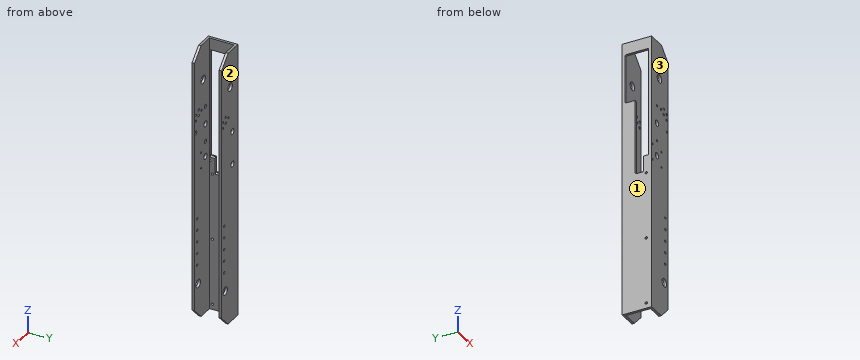
```python
from build123d import *

# Parameters (mm, degrees)
BOSS_EXTRUDE1_DEPTH                                 = 700
CUT_EXTRUDE1_DEPTH                                  = 706.00443261
CHAMFER1_SIZE                                       = 30
SKETCH4_R                                           = 10.5
CUT_EXTRUDE2_DEPTH                                  = 708.990112925
SKETCH5_R                                           = 7.5
CUT_EXTRUDE3_DEPTH                                  = 708.990112925
CHAMFER2_SIZE                                       = 3
FILLET1_R                                           = 3
SKETCH6_R                                           = 3
TENSIONER_HOLES_DEPTH                               = 708.990112925
CSK_FOR_M5_COUNTERSUNK_FLAT_HEAD_SCREW1_D           = 5.8
CSK_FOR_M5_COUNTERSUNK_FLAT_HEAD_SCREW1_DEPTH       = 12
CSK_FOR_M5_COUNTERSUNK_FLAT_HEAD_SCREW1_CSINK_D     = 10.4
CSK_FOR_M5_COUNTERSUNK_FLAT_HEAD_SCREW1_CSINK_ANGLE = 90
CSK_FOR_M5_COUNTERSUNK_FLAT_HEAD_SCREW1_TIP         = 1.742495795
SKETCH11_R                                          = 3
CUT_EXTRUDE4_DEPTH                                  = 10
SKETCH13_R                                          = 2.55
CUT_EXTRUDE5_DEPTH                                  = 10


with BuildPart() as part:
    # Sketch1 → Boss-Extrude1 (new body)
    with BuildSketch(Plane.XY):
        Polygon((0, -37.5), (0, 37.5), (75, 37.5), (75, 31.15), (6.35, 31.15), (6.35, -31.15), (75, -31.15), (75, -37.5), align=None)
    extrude(amount=BOSS_EXTRUDE1_DEPTH)

    # Sketch3 → Cut-Extrude1 (cut, through all)
    with BuildSketch(Plane.ZY):
        Polygon((670.5, -30), (545.5, -30), (395.5, -30), (395.5, -16.85), (355, -16.85), (355, 4.15), (460, 4.15), (545.5, 4.15), (545.5, 30), (670.5, 30), align=None)
    extrude(amount=-CUT_EXTRUDE1_DEPTH, mode=Mode.SUBTRACT)

    # Chamfer1
    chamfer1_edges = [part.edges().sort_by_distance(p)[0] for p in [
        (75, -34.325, 0),
        (75, 34.325, 700),
        (75, -34.325, 700),
        (75, 34.325, 0),
    ]]
    chamfer(chamfer1_edges, length=CHAMFER1_SIZE)

    # Sketch4 → Cut-Extrude2 (cut, through all)
    with BuildSketch(Plane(origin=(0, 37.5, 0), x_dir=(1, 0, 0), z_dir=(0, 1, 0))):
        with Locations(Location((36, -608, 0), (0, 0, 270))):
            Circle(SKETCH4_R)
        with Locations(Location((58.5, -92, 0), (0, 0, 270))):
            Circle(SKETCH4_R)
    extrude(amount=-CUT_EXTRUDE2_DEPTH, mode=Mode.SUBTRACT)

    # Sketch5 → Cut-Extrude3 (cut, through all)
    with BuildSketch(Plane.XZ.offset(37.5)):
        with Locations(Location((25, 487.498060398, 0), (0, 0, 270))):
            Circle(SKETCH5_R)
        with Locations(Location((24.951834767, 403.39807419, 0), (0, 0, 270))):
            Circle(SKETCH5_R)
    extrude(amount=-CUT_EXTRUDE3_DEPTH, mode=Mode.SUBTRACT)

    # Chamfer2
    chamfer2_edges = [part.edges().sort_by_distance(p)[0] for p in [
        (6.35, -23.425, 395.5),
        (6.35, -6.35, 355),
        (6.35, 17.075, 545.5),
    ]]
    chamfer(chamfer2_edges, length=CHAMFER2_SIZE)

    # Fillet1
    fillet1_edges = [part.edges().sort_by_distance(p)[0] for p in [
        (1.675, 4.15, 355),
        (1.675, -16.85, 355),
        (1.675, -30, 395.5),
        (1.675, 30, 545.5),
        (3.175, 30, 670.5),
        (3.175, -30, 670.5),
    ]]
    fillet(fillet1_edges, radius=FILLET1_R)

    # Sketch6 → tensioner holes (cut, through all)
    with BuildSketch(Plane(origin=(0, 37.5, 0), x_dir=(1, 0, 0), z_dir=(0, 1, 0))):
        with Locations(Location((69, -517.498060398, 0), (0, 0, 270))):
            Circle(SKETCH6_R)
        with Locations(Location((69, -532.498060398, 0), (0, 0, 270))):
            Circle(SKETCH6_R)
        with Locations(Location((56.009618943, -524.998060398, 0), (0, 0, 270))):
            Circle(SKETCH6_R)
        with Locations(Location((56.009618943, -539.998060398, 0), (0, 0, 270))):
            Circle(SKETCH6_R)
        with Locations(Location((63, -262, 0), (0, 0, 270))):
            Circle(SKETCH6_R)
        with Locations(Location((63, -232, 0), (0, 0, 270))):
            Circle(SKETCH6_R)
        with Locations(Location((63, -202, 0), (0, 0, 270))):
            Circle(SKETCH6_R)
        with Locations(Location((63, -172, 0), (0, 0, 270))):
            Circle(SKETCH6_R)
        with Locations(Location((63, -142, 0), (0, 0, 270))):
            Circle(SKETCH6_R)
        with Locations(Location((43.019237886, -532.498060398, 0), (0, 0, 270))):
            Circle(SKETCH6_R)
    extrude(amount=-TENSIONER_HOLES_DEPTH, mode=Mode.SUBTRACT)

    # CSK for M5 Countersunk Flat Head Screw1
    with Locations(Plane(origin=(0, -31.15, 0), x_dir=(-1, 0, 0), z_dir=(0, 1, 0))):
        with Locations((-25, 532.573060398), (-25, 442.423060398), (-70.075, 487.498060398)):
            CounterSinkHole(CSK_FOR_M5_COUNTERSUNK_FLAT_HEAD_SCREW1_D / 2, CSK_FOR_M5_COUNTERSUNK_FLAT_HEAD_SCREW1_CSINK_D / 2, depth=CSK_FOR_M5_COUNTERSUNK_FLAT_HEAD_SCREW1_DEPTH, counter_sink_angle=CSK_FOR_M5_COUNTERSUNK_FLAT_HEAD_SCREW1_CSINK_ANGLE)
            with Locations((0, 0, -(CSK_FOR_M5_COUNTERSUNK_FLAT_HEAD_SCREW1_DEPTH + CSK_FOR_M5_COUNTERSUNK_FLAT_HEAD_SCREW1_TIP / 2))):  # 118° drill point
                Cone(0, CSK_FOR_M5_COUNTERSUNK_FLAT_HEAD_SCREW1_D / 2, CSK_FOR_M5_COUNTERSUNK_FLAT_HEAD_SCREW1_TIP, mode=Mode.SUBTRACT)

    # Sketch11 → Cut-Extrude4 (cut)
    with BuildSketch(Plane.ZY):
        with Locations((350, -24)):
            Circle(SKETCH11_R)
        with Locations((13.5, -24)):
            Circle(SKETCH11_R)
        with Locations((181.75, -24)):
            Circle(SKETCH11_R)
    extrude(amount=-CUT_EXTRUDE4_DEPTH, mode=Mode.SUBTRACT)

    # Sketch13 → Cut-Extrude5 (cut)
    with BuildSketch(Plane.XZ.offset(37.5)):
        with Locations(Location((5.152844894, 423.197064064, 0), (0, 0, 270))):
            Circle(SKETCH13_R)
        with Locations(Location((5.152844894, 383.599084317, 0), (0, 0, 270))):
            Circle(SKETCH13_R)
        with Locations(Location((44.75082464, 383.599084317, 0), (0, 0, 270))):
            Circle(SKETCH13_R)
        with Locations(Location((44.75082464, 423.197064064, 0), (0, 0, 270))):
            Circle(SKETCH13_R)
    extrude(amount=-CUT_EXTRUDE5_DEPTH, mode=Mode.SUBTRACT)


solid = part.part
```
Could you check a few things on this model? Use its own coordinates, in mm. Face numbers are marked on the shaded views. Coordinates: 2 decimals unless noted, no trailing zeros. Order: outer loops, then holes, each group sorted by start corner. A loop starts at its lowest first (then second) coordinate and runs counter-clockwise, first axis right, second up. Notation, with made-up numbers: M 59.25,-35.75 L 94.25,-35.75 A19 ccw 94.25,-26.75 Z; hole C 50,76.5 d6. An arc over 180 degrees is marked long. Use a Markdown table: item, result. Add a question column.
Q1. I want a section at B-B on z = 92. List the corners of the cut face in (x, y) for me, then the cut area to 3 significant figures.
Q2. I'm going to push flat-ended pins straight in: pin 1 (18.5 mm diameter, centred on y = 9, z = 229.5, fed in from +X); pin 2 (3.5 mm diameter, centred on x = 69, z = 517.5, fed in from +Y); pin 3 (5 mm diameter, centred on x = 25, z = 442.42, fed in from -Y); pin 4 (6 mm diameter, centred on x = 48.5, y = 29, fed in from +Z). Where does each tip first touch, or does it pass through?
Q3. We'd pull the mould along Y, two halves only. Please class the marked faces 1, 2 and 3: pulls with the +Y half, pulls with the -Y half, needs draft (parallel to the pull), parting line crosses it, or undercut.
Q4. I want a section at A-A on z = 582.5. List the corners of the cut face in (x, y) for me, then the cut area to 3 significant figures.
Q5. If I drill on L1, parallel to Y at x = 35.5, z = 100.5; L2, parallel to Y at x = 3, z = 360.5; L3, parallel to X at y = 24.5, z = 430.5, over which ranges is the centre line in solid material (lowest first)?
Checked values:
| question | item | result |
|---|---|---|
| 1 | outline | M 0,-37.5 L 48,-37.5 L 48,-31.15 L 6.35,-31.15 L 6.35,31.15 L 48,31.15 L 48,37.5 L 0,37.5 Z; M 69,-37.5 L 75,-37.5 L 75,-31.15 L 69,-31.15 Z; M 69,31.15 L 75,31.15 L 75,37.5 L 69,37.5 Z |
| 1 | area | 1,080 mm² |
| 2 | pin 1 | x = 6.35 |
| 2 | pin 2 | through |
| 2 | pin 3 | y = 31.15 |
| 2 | pin 4 | z = 698.59 |
| 3 | face 1 | needs draft |
| 3 | face 2 | pulls with the +Y half |
| 3 | face 3 | pulls with the -Y half |
| 4 | outline | M 0,-37.5 L 75,-37.5 L 75,-31.15 L 6.35,-31.15 L 6.35,-30 L 0,-30 Z; M 0,30 L 6.35,30 L 6.35,31.15 L 75,31.15 L 75,37.5 L 0,37.5 Z |
| 4 | area | 967 mm² |
| 5 | L1 | -37.5 to -31.15, 31.15 to 37.5 |
| 5 | L2 | -37.5 to -16.85, 4.15 to 37.5 |
| 5 | L3 | 0 to 6.35 |
